CAD build for the part. Positions are in the model's coordinates, mm. Coordinates: 2 decimals unless noted, no trailing zeros. Order: outer loops, then holes, each group sorted by start corner. A loop starts at its lowest first (then second) coordinate and runs counter-clockwise, first axis right, second up. Notation, with made-up numbers: M 13.25,8 L 72.25,8 A23 cw 72.25,16 Z; hole C -39.5,73 d5. An arc over 180 degrees is marked long. Write item = value, one per line. Start each with the question number.
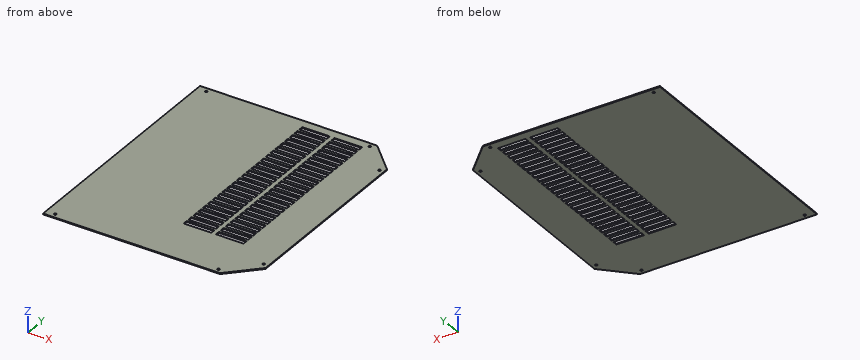
```python
from build123d import *

# Parameters (mm, degrees)
SKETCH_R            = 2.5
PAD_DEPTH           = 2
SKETCH001_W         = 60
SKETCH001_H         = 10
POCKET_DEPTH        = 5
LINEARPATTERN_COUNT = 25
LINEARPATTERN_PITCH = 16.25


with BuildPart() as part:
    # Sketch → Pad (new body)
    with BuildSketch(Plane.XY):
        Polygon((-219.290563, 261.197963), (165.709437, 261.197963), (225.709437, 201.197963), (225.709437, -208.802037), (165.709437, -268.802037), (-219.290563, -268.802037), align=None)
        with Locations((155.709437, 251.197963)):
            Circle(SKETCH_R, mode=Mode.SUBTRACT)
        with Locations((215.709437, 191.197963)):
            Circle(SKETCH_R, mode=Mode.SUBTRACT)
        with Locations((215.709437, -198.802037)):
            Circle(SKETCH_R, mode=Mode.SUBTRACT)
        with Locations((155.709437, -258.802037)):
            Circle(SKETCH_R, mode=Mode.SUBTRACT)
        with Locations((-199.290563, 251.197963)):
            Circle(SKETCH_R, mode=Mode.SUBTRACT)
        with Locations((-199.290563, -258.802037)):
            Circle(SKETCH_R, mode=Mode.SUBTRACT)
    extrude(amount=PAD_DEPTH)

    # Sketch001 → Pocket (cut)
    with BuildSketch(Plane.XY.offset(2)):
        with Locations((45.709437, 236.197963)):
            Rectangle(SKETCH001_W, SKETCH001_H)
        with Locations((115.709437, 236.197963)):
            Rectangle(SKETCH001_W, SKETCH001_H)
    pocket = extrude(amount=-POCKET_DEPTH, mode=Mode.SUBTRACT)

    # LinearPattern: Pocket ×25
    with Locations(*[(0, -i * LINEARPATTERN_PITCH, 0) for i in range(1, LINEARPATTERN_COUNT)]):
        add(pocket, mode=Mode.SUBTRACT)


solid = part.part
```
1. Slice it at A-A (x = 121.5). Give the number of separate pieces and of enclosed holes in the cut face, plus the area to 3 significant figures.
2. Probe L1, parallel to X at y = 92.5, z = 0.7; L2, parallel to X at y = 207, z = 1.1; L3, parallel to X at y = 212.5, z = 1.05. List the from-to ranges inside material, lowest first.
3. Slice it at C-C (x = 172.5). Write the cut outline in (y, z), plus the area to 3 significant figures.
4. Flat gauge pin, fed straight in: pin 1 (4 mm diameter, centred on x = 215.71, y = -198.8, fed in from +Z). Where does the tip first touch, or does it go through?
Calculated:
q1.separate_pieces = 26
q1.enclosed_holes = 0
q1.area = 560 mm²
q2.L1 = -219.29 to 15.71, 75.71 to 85.71, 145.71 to 225.71
q2.L2 = -219.29 to 15.71, 75.71 to 85.71, 145.71 to 219.91
q2.L3 = -219.29 to 214.41
q3.outline = M -262.01,0 L 254.41,0 L 254.41,2 L -262.01,2 Z
q3.area = 1,030 mm²
q4.pin_1 = through
